```python
from build123d import *

# Parameters (mm, degrees)
SKETCH1_R           = 95
BOSS_EXTRUDE1_DEPTH = 20
SKETCH2_R           = 6
CUT_EXTRUDE1_DEPTH  = 20
SKETCH5_R           = 45
BOSS_EXTRUDE3_DEPTH = 55
CUT_EXTRUDE4_DEPTH  = 75


with BuildPart() as part:
    # Sketch1 → Boss-Extrude1 (new body)
    with BuildSketch(Plane.XY):
        Circle(SKETCH1_R)
    extrude(amount=BOSS_EXTRUDE1_DEPTH)

    # Sketch2 → Cut-Extrude1 (cut)
    with BuildSketch(Plane(origin=(0, 0, 0), x_dir=(-1, 0, 0), z_dir=(0, 0, -1))):
        with Locations((0, 70)):
            Circle(SKETCH2_R)
        with Locations((70, 0)):
            Circle(SKETCH2_R)
        with Locations(Location((0, -70, 0), (0, 0, 180))):
            Circle(SKETCH2_R)
        with Locations(Location((-70, 0, 0), (0, 0, 180))):
            Circle(SKETCH2_R)
    extrude(amount=-CUT_EXTRUDE1_DEPTH, mode=Mode.SUBTRACT)

    # Sketch5 → Boss-Extrude3 (add)
    with BuildSketch(Plane.XY.offset(20)):
        Circle(SKETCH5_R)
    extrude(amount=BOSS_EXTRUDE3_DEPTH)

    # Sketch3 → Cut-Extrude4 (cut)
    with BuildSketch(Plane(origin=(0, 0, 0), x_dir=(-1, 0, 0), z_dir=(0, 0, -1))):
        with BuildLine():
            Line((-7, 22.5), (-7, 21.38340478))
            ThreePointArc((-7, 21.38340478), (0, -22.5), (7, 21.38340478))
            Line((7, 21.38340478), (7, 22.5))
            Line((7, 22.5), (7, 25.4))
            Line((7, 25.4), (-7, 25.4))
            Line((-7, 25.4), (-7, 22.5))
        make_face()
    extrude(amount=-CUT_EXTRUDE4_DEPTH, mode=Mode.SUBTRACT)


solid = part.part
```
Verification items for the finished model (mm, model axes). A direction names the side the tool comes from. Coordinates: 2 decimals unless noted, no trailing zeros. Write each loop counter-clockwise with the first axis right and the second up, starting at its lowest first coordinate (ties: lowest second). Pieces come first, ordered by that corner, then holes. Notation, with made-up numbers: M -39.75,-7.5 L 14.25,-7.5 A27 cw 14.25,27.5 Z; hole C 70,83 d1. An arc over 180 degrees is marked long. Answer as a JSON object with one key per item and string values. Group by question number.
(1) Cross-section at D-D, the plane x = 70. Record the cut outline in (y, z).
(2) Cross-section at B-B, the plane x = 0. Record the cut outline in (y, z), and give its area (3 significant figures).
(3) Cross-section at A-A, the plane y = 0. Record the cut outline in (x, z).
(4) Release check for a two-part mould opening along Y. For faces 4 (the face through (20.765, -39.923, 47.115)), 5 (the face through (9, 21, 75)), 6 (the face through (-64, 0, 10)) record: +Y half, -Y half, draft (parallel to the pull), parting line (faces both ways), or undercut.
(5) Gauge pin test, flat ends, axial feed: pin 1 (8 mm diameter, centred on y = 42.5, z = 14.5, fed in from +X); pin 2 (3 mm diameter, centred on x = 15, z = 38, fed in from -Y); pin 3 (1.5 mm diameter, centred on y = 37, z = 9.5, fed in from -X). Record the tip position at first contact, or that the pin passes through.
(6) Cross-section at C-C, the plane z = 55.5. Record the cut outline in (x, y), and give its area (3 significant figures).
(7) Material ranges on line 1 (Y direction, x = -1.5, z = 70.5) (3 decimals); line 2 (Y direction, x = -1, z = 44); line 3 (Z direction, x = 6, y = -72), recorded low to high.
(8) Tool access check on faces 1 (the face through (0, 25.4, 37)), 2 (the face through (41, -20, 20)), 3 (the face through (20, -20, 0)). Record the directions out of +Z, -Z, +X, -X, +Y, -Y that give a thin tool (end or side, any length) a straight path to the whole face; none if there is none.
Reply:
{
 "1": {"outline": "M -64.23,0 L -6,0 L -6,20 L -64.23,20 Z; M 6,0 L 64.23,0 L 64.23,20 L 6,20 Z"},
 "2": {"outline": "M -95,0 L -76,0 L -76,20 L -95,20 Z; M -64,0 L -22.5,0 L -22.5,75 L -45,75 L -45,20 L -64,20 Z; M 25.4,0 L 64,0 L 64,20 L 45,20 L 45,75 L 25.4,75 Z; M 76,0 L 95,0 L 95,20 L 76,20 Z", "area": "4,680 mm²"},
 "3": {"outline": "M -95,0 L -76,0 L -76,20 L -95,20 Z; M -64,0 L -22.5,0 L -22.5,75 L -45,75 L -45,20 L -64,20 Z; M 22.5,0 L 64,0 L 64,20 L 45,20 L 45,75 L 22.5,75 Z; M 76,0 L 95,0 L 95,20 L 76,20 Z"},
 "4": {"face 4": "parting line", "face 5": "draft", "face 6": "undercut"},
 "5": {"pin 1": "x = 86.85", "pin 2": "y = -42.93", "pin 3": "x = -87.81"},
 "6": {"outline": "C 0,0 d90; hole M -7,21.38 A22.5 ccw long 7,21.38 L 7,25.4 L -7,25.4 Z", "area": "4,730 mm²"},
 "7": {"line 1": "-44.975 to -22.45, 25.4 to 44.975", "line 2": "-44.99 to -22.48, 25.4 to 44.99", "line 3": "0 to 20"},
 "8": {"face 1": "+Z, -Z", "face 2": "+Z", "face 3": "-Z, +X, -X, +Y, -Y"}
}
